from build123d import *

# Parameters (mm, degrees)
F1_DEPTH = 1219.2
F2_W     = 25.4
F2_H     = 19.05
F3_DEPTH = 19.051


with BuildPart() as f1:
    # F0 (on Top) → F1 (new body)
    with BuildSketch(Plane.XY):
        Polygon((-31.75, 0), (0, 0), (0, 19.05), (-50.8, 19.05), align=None)
    extrude(amount=-F1_DEPTH)

    # F2 (on face) → F3 (cut, through all)
    with BuildSketch(Plane(origin=(0, 19.05, 0), x_dir=(-1, 0, 0), z_dir=(0, 1, 0))):
        with Locations((12.7, -9.525)):
            Rectangle(F2_W, F2_H)
    extrude(amount=-F3_DEPTH, mode=Mode.SUBTRACT)


solid = f1.part
Geometry check sheet. Reference: the model listing, model coordinates, mm. A direction names the side the tool comes from. Coordinates: 2 decimals unless noted, no trailing zeros. Order: outer loops, then holes, each group sorted by start corner. A loop starts at its lowest first (then second) coordinate and runs counter-clockwise, first axis right, second up. Notation, with made-up numbers: (81, 59) - (102, 59) arc R8 ccw to (102, 69) - close; hole circle Ø5 at (38.25, -2.75). An arc over 180 degrees is marked (long way). Answer in a Markdown table with one row per item. Add a question column.
1) Set-up check for faces 1 (the flat face through (-16, 0, -601)), 2 (the flat face through (-25.4, 10, -10)): record each of +Z, -Z, +X, -X, +Y, -Y from which the full face is reachable in a straight line by a thin tool's end or side.
2) Cross-section at A-A, the plane y = 14.75. Record the cut outline in (x, z), then the cut area to 3 significant figures.
3) Material ranges on line 1 along Z through (x, y) = (-25, 12.75); line 2 along X through (y, z) = (8, -656); line 3 along X through (y, z) = (17.25, -1123), recorded low to high. Write a range as [from, to].
4) Cross-section at B-B, the plane z = -1091.5. Record the cut outline in (x, y), then the cut area to 3 significant figures.
5) Gauge pin test, flat ends, axial feed: P1, Ø8, axis at y = 8, z = -867, coming from the -X side; P2, Ø5.5, axis at x = -17, y = 6, coming from the +Z side; P3, Ø8, axis at y = 10, z = -789, coming from the -X side. Record the tip position at first contact, or that the pin passes through.
6) Cross-section at C-C, the plane x = -14.5. Record the cut outline in (y, z).
Check result:
| question | item | result |
|---|---|---|
| 1 | face 1 | +Z, -Z, +X, -X, -Y |
| 1 | face 2 | +Z, +X, +Y, -Y |
| 2 | outline | (-46.5, -1219.2) - (0, -1219.2) - (0, -19.05) - (-25.4, -19.05) - (-25.4, 0) - (-46.5, 0) - close |
| 2 | area | 56,200 mm² |
| 3 | line 1 | z = [-1219.2, -19.05] |
| 3 | line 2 | x = [-39.75, 0] |
| 3 | line 3 | x = [-49, 0] |
| 4 | outline | (-50.8, 19.05) - (-31.75, 0) - (0, 0) - (0, 19.05) - close |
| 4 | area | 786 mm² |
| 5 | P1 | stops at x = -43.75 |
| 5 | P2 | stops at z = -19.05 |
| 5 | P3 | stops at x = -45.75 |
| 6 | outline | (0, -1219.2) - (19.05, -1219.2) - (19.05, -19.05) - (0, -19.05) - close |
